Could you check a few things on this model? Use its own coordinates, in mm. A direction names the side the tool comes from. Coordinates: 2 decimals unless noted, no trailing zeros. Write each loop counter-clockwise with the first axis right and the second up, starting at its lowest first coordinate (ties: lowest second). Pieces come first, ordered by that corner, then holes.
Item 1: I want a section at B-B on x = 36.5. Please give me the cut outline in (y, z).
Item 2: For P1, Ø2, axis at x = 84, y = -6.5, coming from the -Z side; P2, Ø8, axis at x = 87.5, z = -11, coming from the +Y side; P3, Ø3, axis at x = 63.5, y = -6.5, coming from the -Z side; P4, Ø1.5, axis at x = 37, z = 11, coming from the -Y side, each with a flat end and sliding along its axis, tell me the tip position at first contact or that it passes through.
Item 3: I want a section at A-A on x = 88. Please give me the cut outline in (y, z).
Item 4: Which directions (+Z, -Z, +X, -X, +Y, -Y) give clear straight access to the entire face, cutting with the end or side of a thin tool? Please do faces 1 (the flat face through (85.353, 5.238, 5.369)), 2 (the cylindrical face through (103, -6, 0)), 3 (the flat face through (75, -6, 6)), 4 (the flat face through (85.353, -5.238, -5.369)), 5 (the flat face through (75, 6, -6)).
Item 5: If I drill on probe 1 along Z at (x, y) = (40.5, 0); probe 2 along X at (y, z) = (-11, 9); probe 3 along Z at (x, y) = (12.5, 1), over which ranges is the centre line in solid material (lowest first)?
Autodesk Inventor part; units mm, degrees
ref_plane "YZ Plane" through (0, 0, 0) normal (1, 0, 0) x (0, 1, 0)
ref_plane "XZ Plane" through (0, 0, 0) normal (0, 1, 0) x (-1, 0, 0)
ref_plane "XY Plane" through (0, 0, 0) normal (0, 0, 1) x (1, 0, 0)
sketch "草图1" plane through (0, 0, 0) normal (0, 0, 1) x (1, 0, 0)
  line L0 (0, 29) -> (0, 10)
  line L1 (0, 10) -> (75, 10)
  line L2 (0, 0) -> (110, 0)
  line L3 (110, 0) -> (110, 6)
  line L4 (110, 6) -> (75, 6)
  line L5 (75, 6) -> (75, 10)
  arc A0 (-17.749, 29) -> (-26, 15.7797) centre (14, 0) ccw
  line L6 (0, 29) -> (-17.749, 29)
  line L7 (0, 0) -> (-29, 0)
  line L8 (-26, 15.7797) -> (-26, 0)
  dimension "d0" = 110
  dimension "d1" = 10
  dimension "d2" = 6
  dimension "d4" = 86
  dimension "d5" = 29
  dimension "d8" = 35
  dimension "d14" = 26
  dimension "d15" = 14
revolve "旋转1" add sketch "草图1" angle 360 about axis through (0, 0, 0) along (1, 0, 0)
sketch "草图2" plane through (75, 0, 0) normal (1, 0, 0) x (0, 0, -1)
  circle A0 centre (0, 0) radius 29
  line L0 (0, 10.6066) -> (10.6066, 0)
  line L1 (10.6066, 0) -> (0, -10.6066)
  line L2 (0, -10.6066) -> (-10.6066, 0)
  line L3 (-10.6066, 0) -> (0, 10.6066)
  line L4 (0, 0) -> (0, 10)
  circle A1 centre (0, 0) radius 10
  point P0 (0.6262, 9.9804)
  point P1 (-0.6262, 9.9804)
  point P2 (-9.9804, 0.6262)
  point P3 (-9.9804, -0.6262)
  point P4 (-0.6262, -9.9804)
  point P5 (0.6262, -9.9804)
  point P6 (9.9804, -0.6262)
  point P7 (9.9804, 0.6262)
  dimension "d9" = 7.5
extrude "拉伸1" add sketch "草图2" along normal blind 21 contours L0 A1 L1 L2 L3
thread "螺纹1"
chamfer "倒角1" distance 3 angle 45 1 edges at (0, -10, 0)
properties part number "塞杆" material "不锈钢"
Response values:
1. outline: circle Ø20 at (0, 0)
2. P1: stops at z = -5.11
2. P2: stops at y = 3.61
2. P3: stops at z = -8.66
2. P4: passes through
3. outline: (-9.98, -0.63) - (-0.63, -9.98) arc R10 ccw to (0.63, -9.98) - (9.98, -0.63) arc R10 ccw to (9.98, 0.63) - (0.63, 9.98) arc R10 ccw to (-0.63, 9.98) - (-9.98, 0.63) arc R10 ccw to start
4. face 1: +Z, +X, +Y
4. face 2: +X
4. face 3: +Z, +X, -Y
4. face 4: -Z, +X, -Y
4. face 5: -Z, +X, +Y
5. probe 1: z = -10 to 10
5. probe 2: x = -26 to 0
5. probe 3: z = -9.95 to 9.95
